Part print with two shaded views. Sizes in mm from the minimum x, y, z corner. A direction names the side the tool comes from. Give positions to 0.01 mm unless a question says otherwise; leave off trailing zeros. Write each loop counter-clockwise with the first axis right and the second up, starting at its lowest first coordinate (ties: lowest second). Pieces come first, ordered by that corner, then holes. Notation, with made-up numbers: (35, 65.25) -> (69, 65.25) arc R27 cw to (69, 86.25) -> close; hole circle Ø5 at (65, -17). An arc over 180 degrees is marked (long way). Write item = value, one per line. Start each with the question number.
Q1. Drop flat-ended pins along their axis: P1, Ø18, axis at x = 40, y = 40, coming from the +Z side; P2, Ø3, axis at x = 41.5, y = 50, coming from the +Z side; P3, Ø2, axis at y = 59, z = 9, coming from the +X side; P4, Ø2, axis at x = 24.5, z = 16, coming from the -Y side. Give the stop position or say it passes through.
Q2. Tool access for the marked faces 3 and 4: list every direction of +Z, -Z, +X, -X, +Y, -Y with a clear straight run to the whole face (end or side of a thin tool).
Q3. Saw through at A-A, the plane x = 40. List the corners of the cut face in (y, z), then the cut area to 3 significant figures.
Q4. Wall check: line 1 (Y direction, x = 42, z = 12.25); line 2 (Y direction, x = 40, z = 14.75); line 3 (Z direction, x = 6, y = 23.5). Give the ranges that are in metal, low to high.
Q5. Mould opens along Y. For the marked faces 1 and 2 say: pulls with the +Y half, pulls with the -Y half, needs draft (parallel to the pull), parting line crosses it, or undercut.
Q6. Saw through at D-D, the plane z = 18.25. List the corners of the cut face in (x, y), then the cut area to 3 significant figures.
Q7. Saw through at C-C, the plane z = 5.25. List the corners of the cut face in (x, y).
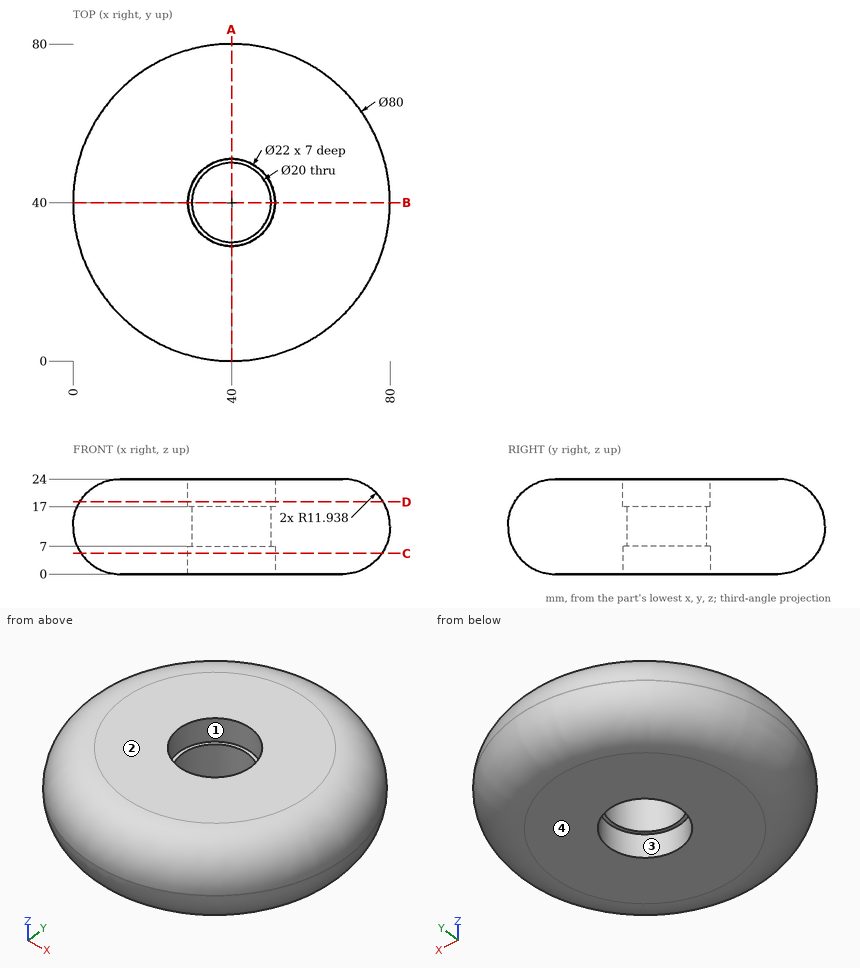
Report:
q1.P1 = through
q1.P2 = 24
q1.P3 = 75.37
q1.P4 = 3.31
q2.face_3 = -Z
q2.face_4 = -Z, +X, -X, +Y, -Y
q3.outline = (0, 11.94) arc R11.94 ccw to (11.94, 0) -> (29, 0) -> (29, 7) -> (30, 7) -> (30, 17) -> (29, 17) -> (29, 24) -> (11.94, 24) arc R11.94 ccw to (0, 12.06) -> close; (50, 7) -> (51, 7) -> (51, 0) -> (68.06, 0) arc R11.94 ccw to (80, 11.94) -> (80, 12.06) arc R11.94 ccw to (68.06, 24) -> (51, 24) -> (51, 17) -> (50, 17) -> close
q3.area = 1,290 mm2
q4.line_1 = 0.05 to 30.2, 49.8 to 79.95
q4.line_2 = 0.31 to 30, 50 to 79.69
q4.line_3 = 5.02 to 18.98
q5.face_1 = undercut
q5.face_2 = needs draft
q6.outline = circle Ø76.54 at (40, 40); hole circle Ø22 at (40, 40)
q6.area = 4,220 mm2
q7.outline = circle Ø75.9 at (40, 40); hole circle Ø22 at (40, 40)
